from build123d import *

# Parameters (mm, degrees)
SKETCH1_W           = 25.4
SKETCH1_H           = 25.4
BOSS_EXTRUDE1_DEPTH = 482.6
SKETCH2_R           = 2.54
CUT_EXTRUDE1_DEPTH  = 2.54


with BuildPart() as part:
    # Sketch1 → Boss-Extrude1 (new body)
    with BuildSketch(Plane(origin=(0, 0, 0), x_dir=(1, 0, 0), z_dir=(0, 1, 0))):
        with Locations((12.7, 12.7)):
            Rectangle(SKETCH1_W, SKETCH1_H)
        Polygon((1.27, 12.361459156), (1.27, 24.13), (12.7, 24.13), (24.13, 24.13), (24.13, 12.7), (24.13, 1.27), (12.7, 1.27), (1.27, 1.27), align=None, mode=Mode.SUBTRACT)
    extrude(amount=BOSS_EXTRUDE1_DEPTH)

    # Sketch2 → Cut-Extrude1 (cut)
    with BuildSketch(Plane(origin=(0, 0, -25.4), x_dir=(-1, 0, 0), z_dir=(0, 0, -1))):
        with Locations((-12.7, 50.874750115)):
            Circle(SKETCH2_R)
    extrude(amount=-CUT_EXTRUDE1_DEPTH, mode=Mode.SUBTRACT)


solid = part.part
Source: CAD feature listing. Evaluate the final solid. Frame: model axes, mm. A direction names the side the tool comes from. Coordinates: 2 decimals unless noted, no trailing zeros. Loops run counter-clockwise (first coordinate to the right, second up) from the corner with the lowest first, then second, coordinate; pieces in that order, holes last. Notation, with made-up numbers: (10.5, 86.5) - (68.5, 86.5) arc R23 ccw to (68.5, 116.5) - close; hole circle Ø2 at (5.25, 13.5). An arc over 180 degrees is marked (long way). One line per question, with ' | ' between items.
1) Pull-direction query (Z, two-part tool) for faces 3 (the face through (13, 238, -25.4)), 4 (the face through (24.13, 238, -13)), 5 (the face through (25.4, 238, -13)); classes: released by +Z, released by -Z, zero draft, split by the parting line, or undercut.
Report:
face 3: released by -Z | face 4: undercut | face 5: zero draft
2) Section B-B, the plane z = -7.25. Return loops of the section in (x, y).
Report:
outline: (0, 0) - (1.27, 0) - (1.27, 482.6) - (0, 482.6) - close; (24.13, 0) - (25.4, 0) - (25.4, 482.6) - (24.13, 482.6) - close
3) Set-up query: faces 1 (the face through (12, 482.6, -1)), 2 (the face through (13, 238, -24.13)). Return all of +Z, -Z, +X, -X, +Y, -Y with unobstructed straight access to the full face (end or side cutting, diameter ignored); none if empty.
Report:
face 1: +Z, -Z, +X, -X, +Y | face 2: +Y, -Y
4) First-contact query: P1, Ø11.5, axis at y = 361, z = -13, coming from the -X side; P2, Ø4, axis at x = 12.7, y = 50.87, coming from the -Z side. Flat tips, straight axial feed; report the tip coordinate or a pass-through.
Report:
P1: stops at x = 0 | P2: stops at z = -1.27
5) Section A-A, the plane y = 320.5. Return loops of the section in (x, z).
Report:
outline: (0, -25.4) - (25.4, -25.4) - (25.4, 0) - (0, 0) - close; hole (1.27, -24.13) - (24.13, -24.13) - (24.13, -1.27) - (1.27, -1.27) - close
6) Line query: line 1 along Z through (x, y) = (7.25, 34); line 2 along X through (y, z) = (140, -5.75); line 3 along Y through (x, z) = (12.7, -25.1). Output: solid intervals per line, ascending.
Report:
line 1: z = -25.4 to -24.13, -1.27 to 0 | line 2: x = 0 to 1.27, 24.13 to 25.4 | line 3: y = 0 to 48.33, 53.41 to 482.6
